Can you work these out from the model? Positions are in its coordinate system, mm. Give positions to 0.01 mm unless a question says otherwise; leave off trailing zeros. Return JSON: item names as keys, results as strings. Group by question number.
Q1. I need wall thicknesses on line 1 along X through (y, z) = (-0.45, 0); line 2 along X through (y, z) = (-0.6, -1); line 3 along Z through (x, y) = (-116.25, -0.2). Which ranges of each line are inside material? Lowest first, please. Write a range as [from, to].
Q2. Will this pin go through, and if not, where does the flat tip stop? pin 1 (2.5 mm diameter, centred on x = -86.25, z = 0, fed in from +Y).
Q3. Suppose I cut it at A-A, the plane y = 0.5. Count the separate pieces of the cut face and the enclosed holes in it, and give its area (3 significant figures).
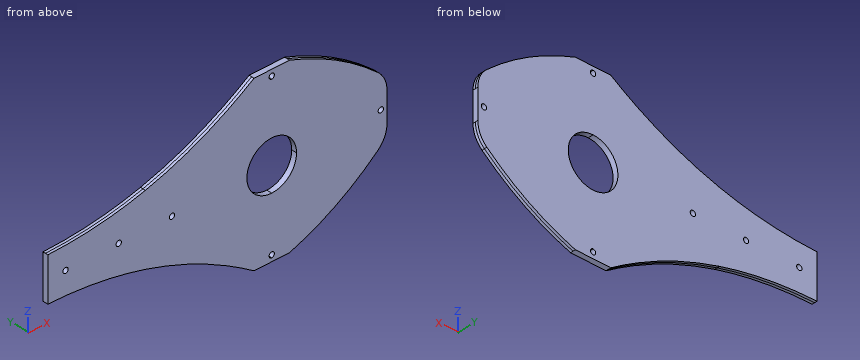
```python
from build123d import *

# Parameters (mm, degrees)
BOSS_EXTRUDE1_DEPTH  = 1.5
SKETCH2_R            = 1.5
CUT_EXTRUDE1_DEPTH   = 82.305365895
FILLET1_R            = 15
FILLET1_OF_MIRROR2_R = 15
BOSS_EXTRUDE2_DEPTH  = 1.5
CUT_EXTRUDE2_DEPTH   = 136.368478737


with BuildPart() as part:
    # Sketch1 → Boss-Extrude1 (new, symmetric)
    with BuildSketch(Plane(origin=(0, 0, 0), x_dir=(1, 0, 0), z_dir=(0, 1, 0))):
        with BuildLine():
            Line((0, 0), (0, 48.75))
            Line((0, 48.75), (10, 48.75))
            add(Edge.make_bspline(
                [(65, 15), (40.796135722, 38.189445994), (10, 48.75)],
                knots=[0, 0, 0, 1, 1, 1], degree=2))
            Line((65, 15), (65, 0))
            Line((65, 0), (0, 0))
        make_face()
    boss_extrude1 = extrude(amount=BOSS_EXTRUDE1_DEPTH, both=True)

    # Sketch2 → Cut-Extrude1 (cut, through all)
    with BuildSketch(Plane(origin=(0, 1.5, 0), x_dir=(1, 0, 0), z_dir=(0, 1, 0))):
        with Locations((0, 45.25)):
            Circle(SKETCH2_R)
        with Locations((61.5, 0)):
            Circle(SKETCH2_R)
    cut_extrude1 = extrude(amount=-CUT_EXTRUDE1_DEPTH, mode=Mode.SUBTRACT)

    # Fillet1
    fillet1_edges = [part.edges().sort_by_distance(p)[0] for p in [
        (65, -0.75, -15),
    ]]
    fillet(fillet1_edges, radius=FILLET1_R)

    # Mirror2: Boss-Extrude1, Cut-Extrude1 across plane
    add(boss_extrude1.mirror(Plane.XY))
    add(cut_extrude1.mirror(Plane.XY), mode=Mode.SUBTRACT)

    # Fillet1 of Mirror2
    fillet1_of_mirror2_edges = [part.edges().sort_by_distance(p)[0] for p in [
        (65, -0.75, 15),
    ]]
    fillet(fillet1_of_mirror2_edges, radius=FILLET1_OF_MIRROR2_R)

    # Sketch3 → Boss-Extrude2 (add, symmetric)
    with BuildSketch(Plane(origin=(0, 0, 0), x_dir=(1, 0, 0), z_dir=(0, 1, 0))):
        with BuildLine():
            Line((-46.25, 0), (0, 0))
            Line((0, 0), (0, 43.75))
            ThreePointArc((0, 43.75), (-1.5, 45.25), (0, 46.75))
            Line((0, 46.75), (0, 48.75))
            Line((0, 48.75), (-10, 48.75))
            add(Edge.make_bspline(
                [(-71.25, 20), (-39.034297028, 28.989339219), (-10, 48.75)],
                knots=[0.450666758, 0.450666758, 0.450666758, 1, 1, 1], degree=2))
            Line((-71.25, 20), (-71.25, 0))
            Line((-71.25, 0), (-57.75, 0))
            ThreePointArc((-57.75, 0), (-56.25, 1.5), (-54.75, 0))
            Line((-54.75, 0), (-46.25, 0))
        make_face()
        with BuildLine():
            Line((-84.75, 0), (-71.25, 0))
            Line((-71.25, 0), (-71.25, 20))
            add(Edge.make_bspline(
                [(-126.25, 12.5), (-97.67939718, 12.625248103), (-71.25, 20)],
                knots=[0, 0, 0, 0.450666758, 0.450666758, 0.450666758], degree=2))
            Line((-126.25, 12.5), (-126.25, 0))
            Line((-126.25, 0), (-117.75, 0))
            ThreePointArc((-117.75, 0), (-116.25, 1.5), (-114.75, 0))
            Line((-114.75, 0), (-87.75, 0))
            ThreePointArc((-87.75, 0), (-86.25, 1.5), (-84.75, 0))
        make_face()
    boss_extrude2 = extrude(amount=BOSS_EXTRUDE2_DEPTH, both=True)

    # Mirror3: Boss-Extrude2 across plane
    add(boss_extrude2.mirror(Plane.XY))

    # Sketch4 → Cut-Extrude2 (cut, through all)
    with BuildSketch(Plane(origin=(0, 1.5, 0), x_dir=(1, 0, 0), z_dir=(0, 1, 0))):
        with BuildLine():
            ThreePointArc((14, 0), (9.899494937, 9.899494937), (0, 14))
            Line((0, 14), (0, -14))
            ThreePointArc((0, -14), (9.899494937, -9.899494937), (14, 0))
        make_face()
        with BuildLine():
            Line((0, -14), (0, 14))
            ThreePointArc((0, 14), (-14, 0), (0, -14))
        make_face()
    extrude(amount=-CUT_EXTRUDE2_DEPTH, mode=Mode.SUBTRACT)


solid = part.part
```
Ans:
{
 "1": {"line 1": "x = [-126.25, -117.75], [-114.75, -87.75], [-84.75, -57.75], [-54.75, -14], [14, 60], [63, 65]", "line 2": "x = [-126.25, -117.37], [-115.13, -87.37], [-85.13, -57.37], [-55.13, -13.96], [13.96, 60.38], [62.62, 65]", "line 3": "z = [-12.77, -1.5], [1.5, 12.77]"},
 "2": {"pin 1": "passes through"},
 "3": {"separate pieces": "1", "enclosed holes": "7", "area": "10,700 mm^2"}
}
